Job drawing, mm, ordinate dimensions from the low corner. One solid piece. Give positions to 0.01 mm unless a question says otherwise; leave off trailing zeros. Loops run counter-clockwise (first coordinate to the right, second up) from the corner with the lowest first, then second, coordinate; pieces in that order, holes last. Notation, with made-up numbers: M -9,16 L 47,16 A24 cw 47,45 Z; hole C 35,18.5 d9. An arc over 180 degrees is marked long. Answer in a Markdown table with one row per item.
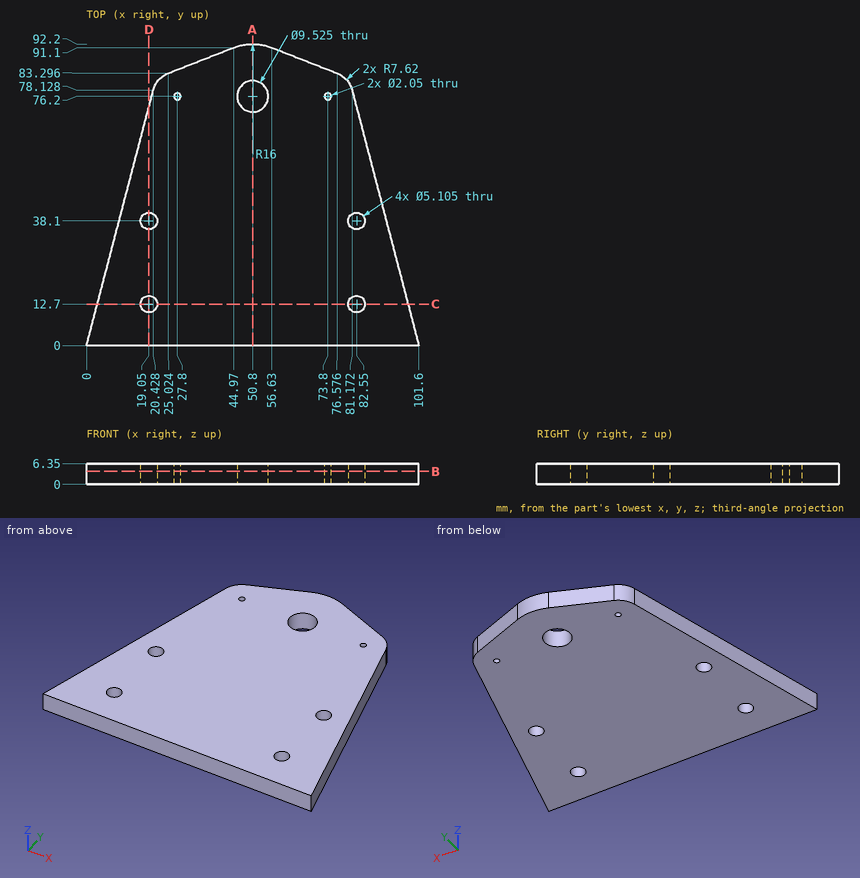
(1) Drill centre lines: line 1 along X through (y, z) = (37.5, 3) (1 decimal); line 2 along X through (y, z) = (36, 1) (1 decimal); line 3 along Y through (x, z) = (27.8, 5) (1 decimal). Where is each one in solid material? Low to high.
Recorded:
| item | result |
|---|---|
| line 1 | x = 9.8 to 16.6, 21.5 to 80.1, 85 to 91.8 |
| line 2 | x = 9.4 to 17.6, 20.5 to 81.1, 84 to 92.2 |
| line 3 | y = 0 to 75.2, 77.2 to 84.4 |
(2) Saw through at B-B (z = 4). Give the number of separate pieces and of enclosed holes in the cut face.
Recorded:
| item | result |
|---|---|
| separate pieces | 1 |
| enclosed holes | 7 |
(3) Pin check, flat tips, straight feed: pin 1 Ø3 at (y, z) = (60.5, 5.5) entering from +X; pin 2 Ø3 at (y, z) = (82.5, 3.5) entering from -X; pin 3 Ø8.5 at (x, y) = (50.8, 76.2) entering from +Z; pin 4 Ø3 at (y, z) = (64, 2) entering from +X. Stop position of each tip, or through.
Recorded:
| item | result |
|---|---|
| pin 1 | stops at x = 86.17 |
| pin 2 | stops at x = 21.88 |
| pin 3 | passes through |
| pin 4 | stops at x = 85.26 |
(4) Saw through at D-D (x = 19.05). Write the cut outline in (y, z), plus the area to 3 significant figures.
Recorded:
| item | result |
|---|---|
| outline | M 0,0 L 10.15,0 L 10.15,6.35 L 0,6.35 Z; M 15.25,0 L 35.55,0 L 35.55,6.35 L 15.25,6.35 Z; M 40.65,0 L 72.86,0 L 72.86,6.35 L 40.65,6.35 Z |
| area | 398 mm^2 |
(5) Saw through at A-A (x = 50.8). Write the cut outline in (y, z).
Recorded:
| item | result |
|---|---|
| outline | M 0,0 L 71.44,0 L 71.44,6.35 L 0,6.35 Z; M 80.96,0 L 92.2,0 L 92.2,6.35 L 80.96,6.35 Z |
(6) Saw through at C-C (y = 12.7). Write the cut outline in (x, z), plus the area to 3 significant figures.
Recorded:
| item | result |
|---|---|
| outline | M 3.32,0 L 16.5,0 L 16.5,6.35 L 3.32,6.35 Z; M 21.6,0 L 80,0 L 80,6.35 L 21.6,6.35 Z; M 85.1,0 L 98.28,0 L 98.28,6.35 L 85.1,6.35 Z |
| area | 538 mm^2 |
